from build123d import *

# Parameters (mm, degrees)
SKETCH1_W           = 5
SKETCH1_H           = 5
BOSS_EXTRUDE1_DEPTH = 675
SKETCH1_3_W         = 5
SKETCH1_3_H         = 10
CUT_EXTRUDE1_DEPTH  = 645
CIRPATTERN1_COUNT   = 4


with BuildPart() as part:
    # Sketch1 → Boss-Extrude1 (new body)
    with BuildSketch(Plane.XY):
        Polygon((-2.5, 10), (-10, 10), (-10, -10), (10, -10), (10, 10), (2.5, 10), (2.5, 5), (-2.5, 5), align=None)
        with Locations((0, 7.5)):
            Rectangle(SKETCH1_W, SKETCH1_H)
    extrude(amount=-BOSS_EXTRUDE1_DEPTH)

    # Sketch1_3 → Cut-Extrude1 (cut)
    with BuildSketch(Plane.XY):
        with Locations((0, 10)):
            Rectangle(SKETCH1_3_W, SKETCH1_3_H)
    cut_extrude1 = extrude(amount=-CUT_EXTRUDE1_DEPTH, mode=Mode.SUBTRACT)

    # CirPattern1: Cut-Extrude1 ×4 about axis
    cirpattern1_axis = Axis((0, 0, 0), (0, 0, 1))
    for i in range(1, CIRPATTERN1_COUNT):
        add(cut_extrude1.rotate(cirpattern1_axis, i * 360 / CIRPATTERN1_COUNT), mode=Mode.SUBTRACT)


solid = part.part
Input: part model. Units: mm. Frame: model coordinates. Coordinates: 2 decimals unless noted, no trailing zeros. Write each loop counter-clockwise with the first axis right and the second up, starting at its lowest first coordinate (ties: lowest second). Pieces come first, ordered by that corner, then holes. Notation, with made-up numbers: M 64.25,78 L 117.25,78 A26 cw 117.25,98 Z; hole C -24,62.25 d4. An arc over 180 degrees is marked long. Answer as a JSON object with one key per item and string values. Group by question number.
(1) Contact query for flat-ended pins moving along their axis: P1, Ø10, axis at y = -2, z = -256.5, coming from the -X side; P2, Ø1.5, axis at y = 1, z = -308.5, coming from the -X side; P3, Ø1.5, axis at x = 7, y = 0.5, coming from the +Z side; P4, Ø2.5, axis at x = 0.5, z = -278, coming from the +Y side. Output: stop coordinate, or through.
(2) Section A-A on z = -578.5. Output: boundary loops of the cut face in (x, y).
(3) Ray query, line 1 along Y through (x, z) = (-6, -592); line 2 along Z through (x, y) = (-8.5, 0.5). Return the intervals inside material, ascending. Write a range as [from, to].
Result set:
{
 "1": {"P1": "stops at x = -10", "P2": "stops at x = -5", "P3": "stops at z = -645", "P4": "stops at y = 5"},
 "2": {"outline": "M -10,-10 L -2.5,-10 L -2.5,-5 L 2.5,-5 L 2.5,-10 L 10,-10 L 10,-2.5 L 5,-2.5 L 5,2.5 L 10,2.5 L 10,10 L 2.5,10 L 2.5,5 L -2.5,5 L -2.5,10 L -10,10 L -10,2.5 L -5,2.5 L -5,-2.5 L -10,-2.5 Z"},
 "3": {"line 1": "y = [-10, -2.5], [2.5, 10]", "line 2": "z = [-675, -645]"}
}
